Build history of the part. All positions in model axes, mm. A direction names the side the tool comes from. Coordinates: 2 decimals unless noted, no trailing zeros. Order: outer loops, then holes, each group sorted by start corner. A loop starts at its lowest first (then second) coordinate and runs counter-clockwise, first axis right, second up. Notation, with made-up numbers: (50.5, 45.5) - (71.5, 45.5) arc R27 ccw to (71.5, 62.5) - close; hole circle Ø7 at (25.5, 21). An arc over 180 degrees is marked (long way). Return JSON: item names as keys, results as strings.
from build123d import *

# Parameters (mm, degrees)
SKETCH_1_W                 = 14.1
SKETCH_1_H                 = 31.1
SKETCH_1_R                 = 1.4
EXTRUDE_1_DEPTH            = 1.6
SKETCH_2_R                 = 2.9
EXTRUDE_2_DEPTH            = 1
SKETCH_3_R                 = 2.4
EXTRUDE_3_DEPTH            = 8
FILLET_1_R                 = 2.4
FILLET_1_OF_MIRROR_1_R     = 2.4
SKETCH_4_W                 = 7
SKETCH_4_H                 = 7
EXTRUDE_4_DEPTH            = 5.2
SKETCH_5_W                 = 2.5
SKETCH_5_H                 = 2.5
EXTRUDE_5_DEPTH            = 2.5
EXTRUDE_6_DEPTH            = 0.3
PATTERN_LINEAR_1_COUNT     = 2
PATTERN_LINEAR_1_PITCH     = 2.5
PATTERN_LINEAR_1_COL_COUNT = 2
PATTERN_LINEAR_1_COL_PITCH = 2.5


with BuildPart() as part:
    # 草图1 → 凸台-拉伸1 (new body)
    with BuildSketch(Plane(origin=(0, 0, 0), x_dir=(1, 0, 0), z_dir=(0, 1, 0))):
        Rectangle(SKETCH_1_W, SKETCH_1_H)
        with Locations((0, 8.65)):
            Circle(SKETCH_1_R, mode=Mode.SUBTRACT)
    extrude(amount=EXTRUDE_1_DEPTH)

    # 草图2 → 凸台-拉伸2 (add)
    with BuildSketch(Plane.XY.offset(15.55)):
        with Locations((-3.5, 3.7)):
            Circle(SKETCH_2_R)
    extrude_2 = extrude(amount=EXTRUDE_2_DEPTH)

    # 草图3 → 凸台-拉伸3 (add)
    with BuildSketch(Plane.XY.offset(16.55)):
        with Locations((-3.5, 3.7)):
            Circle(SKETCH_3_R)
    extrude_3 = extrude(amount=EXTRUDE_3_DEPTH)

    # 圆角1
    fillet_1_edges = [part.edges().sort_by_distance(p)[0] for p in [
        (-5.9, 3.7, 24.55),
    ]]
    fillet(fillet_1_edges, radius=FILLET_1_R)

    # 镜向1: 凸台-拉伸2, 凸台-拉伸3 across plane
    add(extrude_2.mirror(Plane(origin=(0, 0, 0), x_dir=(0, 0, 1), z_dir=(1, 0, 0))))
    add(extrude_3.mirror(Plane(origin=(0, 0, 0), x_dir=(0, 0, 1), z_dir=(1, 0, 0))))

    # 圆角1 of 镜向1
    fillet_1_of_mirror_1_edges = [part.edges().sort_by_distance(p)[0] for p in [
        (5.9, 3.7, 24.55),
    ]]
    fillet(fillet_1_of_mirror_1_edges, radius=FILLET_1_OF_MIRROR_1_R)

    # 草图4 → 凸台-拉伸4 (add)
    with BuildSketch(Plane(origin=(0, 1.6, 0), x_dir=(1, 0, 0), z_dir=(0, 1, 0))):
        with Locations((-3.95, -0.45)):
            Rectangle(SKETCH_4_W, SKETCH_4_H)
    extrude(amount=EXTRUDE_4_DEPTH)

    # 草图5 → 凸台-拉伸5 (add)
    with BuildSketch(Plane(origin=(0, 1.6, 0), x_dir=(1, 0, 0), z_dir=(0, 1, 0))):
        with Locations((0, 13.8)):
            Rectangle(SKETCH_5_W, SKETCH_5_H)
    extrude_5 = extrude(amount=EXTRUDE_5_DEPTH)

    # 草图6 → 凸台-拉伸6 (add, symmetric)
    with BuildSketch(Plane(origin=(0, 0, 0), x_dir=(0, 0, -1), z_dir=(1, 0, 0))):
        with BuildLine():
            Line((13.5, -0.5), (13.5, 5.7))
            ThreePointArc((13.5, 5.7), (13.792893219, 6.407106781), (14.5, 6.7))
            Line((14.5, 6.7), (21.3, 6.7))
            Line((21.3, 6.7), (21.3, 6.1))
            Line((21.3, 6.1), (14.5, 6.1))
            ThreePointArc((14.5, 6.1), (14.217157288, 5.982842712), (14.1, 5.7))
            Line((14.1, 5.7), (14.1, -0.5))
            Line((14.1, -0.5), (13.5, -0.5))
        make_face()
    extrude_6 = extrude(amount=EXTRUDE_6_DEPTH, both=True)

    # 阵列(线性)1: 凸台-拉伸5, 凸台-拉伸6 ×2
    with Locations(*[(-i * PATTERN_LINEAR_1_PITCH, 0, 0) for i in range(1, PATTERN_LINEAR_1_COUNT)]):
        add(extrude_5)
        add(extrude_6)

    # 阵列(线性)1 col: 凸台-拉伸5, 凸台-拉伸6 ×2
    with Locations(*[(i * PATTERN_LINEAR_1_COL_PITCH, 0, 0) for i in range(1, PATTERN_LINEAR_1_COL_COUNT)]):
        add(extrude_5)
        add(extrude_6)


solid = part.part
1. Drop flat-ended pins along their axis: pin 1 (2 mm diameter, centred on x = -5.5, y = 0.5, fed in from -Z); pin 2 (4.5 mm diameter, centred on x = 0, z = -8.65, fed in from +Y); pin 3 (3 mm diameter, centred on y = 3, z = 5.5, fed in from -X); pin 4 (0.8 mm diameter, centred on y = 5, z = -17, fed in from +X). Give the stop position or say it passes through.
Check values:
{"pin 1": "z = -15.55", "pin 2": "y = 1.6", "pin 3": "x = -7.05", "pin 4": "through"}
2. Probe L1, parallel to X at y = 1.05, z = -8.65; L2, parallel to Z at x = 0, y = 0.35; L3, parallel to Z at x = -1.75, y = 3. List the from-to ranges inside material, lowest first.
Check values:
{"L1": "-7.05 to -1.4, 1.4 to 7.05", "L2": "-15.55 to -10.05, -7.25 to 15.55", "L3": "-15.05 to -12.55, -3.05 to 3.95, 15.55 to 23.64"}
3. Cut at D-D on x = -4.5. Give the cut face in (y, z), plus the area to 3 significant figures.
Check values:
{"outline": "(0, -15.55) - (1.6, -15.55) - (1.6, -3.05) - (6.8, -3.05) - (6.8, 3.95) - (1.6, 3.95) - (1.6, 15.55) - (6.42, 15.55) - (6.42, 16.55) - (5.88, 16.55) - (5.88, 22.15) arc R2.18 ccw to (1.52, 22.15) - (1.52, 16.55) - (0.98, 16.55) - (0.98, 15.55) - (0, 15.55) - close", "area": "124 mm²"}
4. Cut at A-A on z = -8.65. Give the cut face in (x, y).
Check values:
{"outline": "(-7.05, 0) - (-1.4, 0) - (-1.4, 1.6) - (-7.05, 1.6) - close; (1.4, 0) - (7.05, 0) - (7.05, 1.6) - (1.4, 1.6) - close"}
5. Cut at C-C on z = -2. Give the cut face in (x, y), plus the area to 3 significant figures.
Check values:
{"outline": "(-7.45, 1.6) - (-7.05, 1.6) - (-7.05, 0) - (7.05, 0) - (7.05, 1.6) - (-0.45, 1.6) - (-0.45, 6.8) - (-7.45, 6.8) - close", "area": "59.0 mm²"}
6. Mould opens along Z. For faces 6 (the cylindrical face through (0.004, 6.399, -13.785)), 7 (the flat face through (7.05, 1, 0)), 8 (the cylindrical face through (2.504, 6.399, -13.785)) say: pulls with the +Z half, pulls with the -Z half, needs draft (parallel to the pull), parting line crosses it, or undercut.
Check values:
{"face 6": "pulls with the +Z half", "face 7": "needs draft", "face 8": "undercut"}
7. Tool access for faces 1 (the flat face through (-2.8, 6.4, -16.8)), 2 (the flat face through (0.3, 6.4, -16.8)), 3 (the flat face through (0, 3, -15.05)), 4 (the flat face through (-4, 4, -3.05)), 5 (the flat face through (5, 6, 16.55)): list every direction of +Z, -Z, +X, -X, +Y, -Y with a clear straight run to the whole face (end or side of a thin tool).
Check values:
{"face 1": "-Z, -X, +Y", "face 2": "+Z, -Z, +Y", "face 3": "-Z, +X, -X", "face 4": "+X, -X, +Y", "face 5": "+Z"}
8. Cut at B-B on y = 3.7. Give the cut face in (x, z).
Check values:
{"outline": "(-7.45, -3.05) - (-0.45, -3.05) - (-0.45, 3.95) - (-7.45, 3.95) - close; (-6.4, 15.55) - (-0.6, 15.55) - (-0.6, 16.55) - (-1.1, 16.55) - (-1.1, 22.15) arc R2.4 ccw to (-5.9, 22.15) - (-5.9, 16.55) - (-6.4, 16.55) - close; (-3.75, -15.05) - (3.75, -15.05) - (3.75, -12.55) - (-3.75, -12.55) - close; (0.6, 15.55) - (6.4, 15.55) - (6.4, 16.55) - (5.9, 16.55) - (5.9, 22.15) arc R2.4 ccw to (1.1, 22.15) - (1.1, 16.55) - (0.6, 16.55) - close"}
